from build123d import *

# Parameters (mm, degrees)
F0_W       = 58
F0_H       = 12
F1_DEPTH   = 3.5
F2_W       = 14
F2_H       = 5
F2_W_2     = 6
F2_H_2     = 1.5
F3_DEPTH   = 8.5
F4_R       = 5
F5_SIZE2   = 1.0919107028
F5_SIZE    = 3
F5_2_SIZE2 = 1.0919107028
F5_2_SIZE  = 3
F6_R       = 0.7
F7_R       = 0.3


with BuildPart() as f1:
    # F0 (on Top) → F1 (new body)
    with BuildSketch(Plane.XY):
        Rectangle(F0_W, F0_H)
    extrude(amount=F1_DEPTH)

    # F2 (on Right) → F3 (cut, symmetric)
    with BuildSketch(Plane.YZ):
        with Locations((0, 1.75)):
            Rectangle(F2_W, F2_H)
        with Locations((0, 1.75)):
            Rectangle(F2_W_2, F2_H_2, mode=Mode.SUBTRACT)
    extrude(amount=F3_DEPTH, both=True, mode=Mode.SUBTRACT)

    # F4
    f4_edges = [f1.edges().sort_by_distance(p)[0] for p in [
        (29, -6, 1.75),
        (29, 6, 1.75),
        (-29, -6, 1.75),
        (-29, 6, 1.75),
    ]]
    fillet(f4_edges, radius=F4_R)

    # F5
    f5_edges = [f1.edges().sort_by_distance(p)[0] for p in [
        (16.25, -6, 3.5),
    ]]
    f5_side = f1.faces().sort_by_distance((18.333459, 0, 3.5))[0]
    chamfer(f5_edges, length=F5_SIZE, length2=F5_SIZE2, reference=f5_side)

    # F5#2
    f5_2_edges = [f1.edges().sort_by_distance(p)[0] for p in [
        (-16.25, -6, 3.5),
    ]]
    f5_2_side = f1.faces().sort_by_distance((-18.333459, 0, 3.5))[0]
    chamfer(f5_2_edges, length=F5_2_SIZE, length2=F5_2_SIZE2, reference=f5_2_side)

    # F6
    f6_edges = [f1.edges().sort_by_distance(p)[0] for p in [
        (0, 3, 2.5),
        (0, -3, 2.5),
        (0, -3, 1),
        (0, 3, 1),
    ]]
    fillet(f6_edges, radius=F6_R)

    # F7
    f7_edges = [f1.edges().sort_by_distance(p)[0] for p in [
        (8.5, 0, 2.5),
        (-8.5, 0, 2.5),
        (-8.5, 0, 3.5),
        (-8.5, -4.5, 2.954045),
        (-8.5, -6, 1.204045),
        (-8.5, 4.5, 2.954045),
        (-8.5, 6, 1.204045),
        (8.5, 6, 1.204045),
        (8.5, 4.5, 2.954045),
        (8.5, 0, 3.5),
        (8.5, -4.5, 2.954045),
        (8.5, -6, 1.204045),
        (16.25, -6, 2.408089),
        (25.414214, -2.414214, 3.5),
        (-25.414214, -2.414214, 3.5),
        (-27.535534, -4.535534, 2.408089),
    ]]
    fillet(f7_edges, radius=F7_R)


solid = f1.part
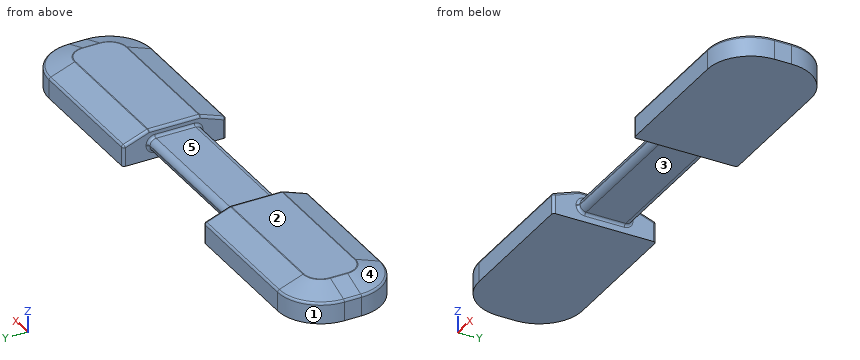
Verification items for the finished model (mm, model axes). Face numbers are marked on the shaded views. A direction names the side the tool comes from. Give positions to 0.01 mm unless a question says otherwise; leave off trailing zeros. Write each loop counter-clockwise with the first axis right and the second up, starting at its lowest first coordinate (ties: lowest second). Pieces come first, ordered by that corner, then holes. Notation, with made-up numbers: (89, 84) - (140, 84) arc R23 cw to (140, 112) - close; hole circle Ø9 at (15, 59.25). An arc over 180 degrees is marked (long way). Answer as CSV lines item,"result". Start each with the question number.
1. Sectioned sample at C-C (x = -7.5). Record the boundary of the cut face in (y, z).
2. Set-up check for the marked faces 4 and 5: record each of +Z, -Z, +X, -X, +Y, -Y from which the full face is reachable in a straight line by a thin tool's end or side.
3. Depth check by flat-ended pin: pin 1 (1.4 mm diameter, centred on x = 3.5, y = 1, fed in from +Z); pin 2 (1.4 mm diameter, centred on x = 3.5, y = 0, fed in from -Z). Enter the tip coordinate at first touch or a pass-through.
4. Thickness scan on line 1 (Z direction, x = -9.5, y = -4.25); line 2 (X direction, y = 4.75, z = 0.15); line 3 (X direction, y = 3.5, z = 2.4). Record the ranges inside material, lowest first.
5. Draft check along X on the marked faces 1, 2 and 3. Enter one of: pulls with the +X half, pulls with the -X half, needs draft (parallel to the pull), parting line crosses it, or undercut.
6. Sectioned sample at A-A (x = 11). Record the boundary of the cut face in (y, z).
7. Sectioned sample at B-B (y = 0.5). Record the boundary of the cut face in (x, z).
Derived:
1,outline,"(-3, 1.7) arc R0.7 ccw to (-2.3, 1) - (2.3, 1) arc R0.7 ccw to (3, 1.7) - (3, 1.8) arc R0.7 ccw to (2.3, 2.5) - (-2.3, 2.5) arc R0.7 ccw to (-3, 1.8) - close"
2,face 4,"+Z, -X, -Y"
2,face 5,"+Z, +Y, -Y"
3,pin 1,"z = 2.5"
3,pin 2,"z = 1"
4,line 1,"0 to 3.05"
4,line 2,"-27.31 to -8.5, 8.5 to 27.31"
4,line 3,"-28.24 to -8.5, 8.5 to 28.24"
5,face 1,"pulls with the -X half"
5,face 2,"needs draft"
5,face 3,"undercut"
6,outline,"(-6, 0) - (6, 0) - (6, 2.2) arc R0.3 ccw to (5.8, 2.48) - (3.05, 3.48) arc R0.3 ccw to (2.95, 3.5) - (-2.95, 3.5) arc R0.3 ccw to (-3.05, 3.48) - (-5.8, 2.48) arc R0.3 ccw to (-6, 2.2) - close"
7,outline,"(-29, 0) - (-8.5, 0) - (-8.5, 0.7) arc R0.3 cw to (-8.2, 1) - (8.2, 1) arc R0.3 cw to (8.5, 0.7) - (8.5, 0) - (29, 0) - (29, 2.2) arc R0.3 ccw to (28.8, 2.48) - (26.05, 3.48) arc R0.3 ccw to (25.95, 3.5) - (8.8, 3.5) arc R0.3 ccw to (8.5, 3.2) - (8.5, 2.8) arc R0.3 cw to (8.2, 2.5) - (-8.2, 2.5) arc R0.3 cw to (-8.5, 2.8) - (-8.5, 3.2) arc R0.3 ccw to (-8.8, 3.5) - (-25.95, 3.5) arc R0.3 ccw to (-26.05, 3.48) - (-28.8, 2.48) arc R0.3 ccw to (-29, 2.2) - close"
